from build123d import *

# Parameters (mm, degrees)
CYLINDER_R     = 1.5
CYLINDER_DEPTH = 22


with BuildPart() as cylinder:
    # Cylinder → Cylinder (new body)
    with BuildSketch(Plane(origin=(0, 18, -11), x_dir=(1, 0, 0), z_dir=(0, 0, 1))):
        Circle(CYLINDER_R)
    extrude(amount=CYLINDER_DEPTH)


with BuildPart() as cut:
    # Sketch → Revolve (revolve)
    with BuildSketch(Plane.XY):
        Polygon((4.05, 0), (4.05, 18), (10.05, 18), (10.05, 8.389587), (40, 8.389587), (31.909247, 5.444793), (31.909247, 2.944793), (40, 0), align=None)
    revolve(axis=Axis((0, 0, 0), (0, 1, 0)))

    # Cut: cut Cylinder
    add(cylinder.part, mode=Mode.SUBTRACT)


solid = cut.part
CAD build for the part. Positions are in the model's coordinates, mm. A direction names the side the tool comes from. Round coordinates to 2 decimals unless told otherwise and drop trailing zeros. Write each loop counter-clockwise with the first axis right and the second up, starting at its lowest first coordinate (ties: lowest second). Pieces come first, ordered by that corner, then holes.
(1) Drop flat-ended pins along their axis: P1, Ø8, axis at y = 14, z = -9.5, coming from the +X side; P2, Ø10, axis at x = 2.5, y = 8.5, coming from the -Z side. Give the stop position or say it passes through.
(2) 3-axis set-ups, long thin cutter, end or side, ignore diameter. For faces 1 (the face through (-32.3, 5.6, -1.4)), 2 (the face through (-8, 8.39, 8)), 3 (the face through (8, 0, -1)): which of +Z, -Z, +X, -X, +Y, -Y reach the whole face in a straight line?
(3) Slice it at A-A, the plane x = 0. Write the cut outline in (y, z), and give its area (3 significant figures).
(4) Slice it at D-D, the plane y = 4. Write the cut outline in (x, z).
(5) Slice it at B-B, the plane z = 0. Write the cut outline in (x, y).
(6) Probe line 1 along Z through (x, y) = (0, 14); line 2 along Z through (x, y) = (0, 4); line 3 along Y through (x, z) = (-8.5, 13). List the from-to ranges inside material, lowest first.
(7) Mould opens along Z. For faces 4 (the face through (30.436, 4.177, -9.585)), 5 (the face through (3.74, 9.13, 1.55)), 6 (the face through (6, 18, 0)) say: pulls with the +Z half, pulls with the -Z half, needs draft (parallel to the pull), parting line crosses it, or undercut.
(8) Slice it at C-C, the plane y = 10.75. Write the cut outline in (x, z).
From the geometry:
1. P1: stops at x = 8.41
1. P2: stops at z = -40
2. face 1: none
2. face 2: +Y
2. face 3: +Z, -Z, +X, -X, -Y
3. outline: (0, -40) - (2.94, -31.91) - (5.44, -31.91) - (8.39, -40) - (8.39, -10.05) - (16.5, -10.05) - (16.5, -4.05) - (0, -4.05) - close; (0, 4.05) - (16.5, 4.05) - (16.5, 10.05) - (8.39, 10.05) - (8.39, 40) - (5.44, 31.91) - (2.94, 31.91) - (0, 40) - close
3. area: 612 mm2
4. outline: circle Ø63.82 at (0, 0); hole circle Ø8.1 at (0, 0)
5. outline: (-40, 0) - (-4.05, 0) - (-4.05, 18) - (-10.05, 18) - (-10.05, 8.39) - (-40, 8.39) - (-31.91, 5.44) - (-31.91, 2.94) - close; (4.05, 0) - (40, 0) - (31.91, 2.94) - (31.91, 5.44) - (40, 8.39) - (10.05, 8.39) - (10.05, 18) - (4.05, 18) - close
6. line 1: z = -10.05 to -4.05, 4.05 to 10.05
6. line 2: z = -31.91 to -4.05, 4.05 to 31.91
6. line 3: y = 0 to 8.39
7. face 4: parting line crosses it
7. face 5: undercut
7. face 6: needs draft
8. outline: circle Ø20.1 at (0, 0); hole circle Ø8.1 at (0, 0)
